Input: part model. Units: mm. Frame: model coordinates. Give positions to 0.01 mm unless a question says otherwise; leave off trailing zeros. Loops run counter-clockwise (first coordinate to the right, second up) from the corner with the lowest first, then second, coordinate; pieces in that order, holes last. Notation, with made-up numbers: (-17.75, 52.5) - (-2.75, 52.5) arc R20 cw to (-2.75, 73.5) - close; hole circle Ø2 at (-33.5, -29.5). An arc over 180 degrees is marked (long way). One line per item, written item: value.
from build123d import *

# Parameters (mm, degrees)
F1_DEPTH = 7.5
F2_R     = 11.50533
F3_DEPTH = 25
F4_R     = 3
F5_DEPTH = 25
F6_R     = 3
F7_DEPTH = 25


with BuildPart() as f1:
    # F0 (on Front) → F1 (new body)
    with BuildSketch(Plane.XZ):
        Polygon((45.799506, 0), (0, 56.201915), (-45.799506, 0), (0, -56.201915), align=None)
    extrude(amount=F1_DEPTH)

    # F2 (on face) → F3 (cut)
    with BuildSketch(Plane.XZ.offset(7.5)):
        Circle(F2_R)
    extrude(amount=-F3_DEPTH, mode=Mode.SUBTRACT)

    # F4 (on face) → F5 (cut)
    with BuildSketch(Plane.XZ.offset(7.5)):
        with Locations((0, 47.198402)):
            Circle(F4_R)
    extrude(amount=-F5_DEPTH, mode=Mode.SUBTRACT)

    # F6 (on face) → F7 (cut)
    with BuildSketch(Plane(origin=(0, 0, 0), x_dir=(-1, 0, 0), z_dir=(0, 1, 0))):
        with Locations((0, -41.517954)):
            Circle(F6_R)
    extrude(amount=-F7_DEPTH, mode=Mode.SUBTRACT)


solid = f1.part
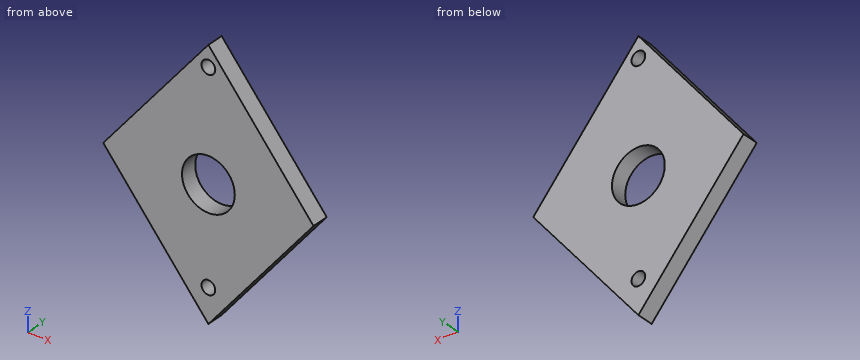
Item 1: Section B-B, the plane y = -6. Output: boundary loops of the cut face in (x, z), and give its area (3 significant figures).
Verdict:
outline: (-45.8, 0) - (0, -56.2) - (45.8, 0) - (0, 56.2) - close; hole circle Ø23.01 at (0, 0); hole circle Ø6 at (0, -41.52); hole circle Ø6 at (0, 47.2)
area: 4,680 mm^2
Item 2: Material intervals for L1, parallel to Z at x = 0, y = -4; L2, parallel to Z at x = 6.5, y = -0.75; L3, parallel to Z at x = 5.5, y = -2.25, sorted ascending.
Verdict:
L1: z = -56.2 to -44.52, -38.52 to -11.51, 11.51 to 44.2, 50.2 to 56.2
L2: z = -48.23 to -9.49, 9.49 to 48.23
L3: z = -49.45 to -10.11, 10.11 to 49.45
Item 3: Section C-C, the plane x = -30.5. Output: boundary loops of the cut face in (y, z).
Verdict:
outline: (-7.5, -18.77) - (0, -18.77) - (0, 18.77) - (-7.5, 18.77) - close
Item 4: Section D-D, the plane z = 30.5. Output: boundary loops of the cut face in (x, y).
Verdict:
outline: (-20.94, -7.5) - (20.94, -7.5) - (20.94, 0) - (-20.94, 0) - close
Item 5: Pin query (flat end, axial travel): P1, Ø2, axis at x = -3.5, y = -2.5, coming from the -Z side; P2, Ø4, axis at x = 7, z = 24.5, coming from the +Y side; P3, Ø3, axis at x = -0.5, y = -3, coming from the -Z side; P4, Ø1, axis at x = 14.5, y = -6.5, coming from the -Z side. Return the tip coordinate at first contact, or that it passes through.
Verdict:
P1: stops at z = -53.13
P2: stops at y = 0
P3: stops at z = -56.2
P4: stops at z = -39.02
Item 6: Section A-A, the plane z = 9. Output: boundary loops of the cut face in (x, y), and give its area (3 significant figures).
Verdict:
outline: (-38.47, -7.5) - (-7.17, -7.5) - (-7.17, 0) - (-38.47, 0) - close; (7.17, -7.5) - (38.47, -7.5) - (38.47, 0) - (7.17, 0) - close
area: 469 mm^2
